Verification items for the finished model (mm, model axes). A direction names the side the tool comes from. Round coordinates to 2 decimals unless told otherwise and drop trailing zeros. Loops run counter-clockwise (first coordinate to the right, second up) from the corner with the lowest first, then second, coordinate; pieces in that order, holes last. Notation, with made-up numbers: M 38.25,36 L 57.25,36 A30 cw 57.25,67 Z; hole C 50,57 d5. An arc over 180 degrees is marked long. Answer as CSV lines item,"result".
Autodesk Inventor part; units mm, degrees
ref_plane "YZ Plane" through (0, 0, 0) normal (1, 0, 0) x (0, 1, 0)
ref_plane "XZ Plane" through (0, 0, 0) normal (0, 1, 0) x (-1, 0, 0)
ref_plane "XY Plane" through (0, 0, 0) normal (0, 0, 1) x (1, 0, 0)
sketch "Sketch1" plane through (0, 0, 0) normal (0, 0, 1) x (1, 0, 0)
  line L0 (0, 0) -> (180, 0)
  line L1 (180, 0) -> (180, -10)
  line L2 (180, -10) -> (0, -10)
  line L3 (0, -10) -> (0, 0)
  line L4 (5.5, 0) -> (24.5, 0)
  line L5 (24.5, 0) -> (24.5, 4.5)
  line L6 (24.5, 4.5) -> (5.5, 4.5)
  line L7 (5.5, 4.5) -> (5.5, 0)
  line L8 (54.5, 4.5) -> (35.5, 4.5)
  line L9 (54.5, 0) -> (54.5, 4.5)
  line L10 (35.5, 4.5) -> (35.5, 0)
  line L11 (84.5, 4.5) -> (65.5, 4.5)
  line L12 (84.5, 0) -> (84.5, 4.5)
  line L13 (65.5, 4.5) -> (65.5, 0)
  line L14 (114.5, 4.5) -> (95.5, 4.5)
  line L15 (114.5, 0) -> (114.5, 4.5)
  line L16 (95.5, 4.5) -> (95.5, 0)
  line L17 (144.5, 4.5) -> (125.5, 4.5)
  line L18 (144.5, 0) -> (144.5, 4.5)
  line L19 (125.5, 4.5) -> (125.5, 0)
  line L20 (174.5, 4.5) -> (155.5, 4.5)
  line L21 (174.5, 0) -> (174.5, 4.5)
  line L22 (155.5, 4.5) -> (155.5, 0)
  dimension "d0" = 180
  dimension "d1" = 10
  dimension "d2" = 19
  dimension "d3" = 4.5
  dimension "d4" = 5.5
  dimension "d7" = 30
extrude "Extrusion1" add sketch "Sketch1" along normal blind 3
properties part number "tray_side_support"
1) Draft check along X on faces 4 (the flat face through (174.5, 2, 1)), 5 (the flat face through (5.5, 2, 1)), 6 (the flat face through (120, 0, 1)). Enter one of: +X half, -X half, draft (parallel to the pull), parting line (faces both ways), or undercut.
Here are the results:
face 4,"+X half"
face 5,"-X half"
face 6,"undercut"
2) Section check C-C (x = 121.5). Record the cut outline in (y, z).
Here are the results:
outline,"M -10,0 L 0,0 L 0,3 L -10,3 Z"
3) Section check A-A (y = 2.5). Record the cut outline in (x, z), plus the area to 3 significant figures.
Here are the results:
outline,"M 5.5,0 L 24.5,0 L 24.5,3 L 5.5,3 Z; M 35.5,0 L 54.5,0 L 54.5,3 L 35.5,3 Z; M 65.5,0 L 84.5,0 L 84.5,3 L 65.5,3 Z; M 95.5,0 L 114.5,0 L 114.5,3 L 95.5,3 Z; M 125.5,0 L 144.5,0 L 144.5,3 L 125.5,3 Z; M 155.5,0 L 174.5,0 L 174.5,3 L 155.5,3 Z"
area,"342 mm^2"
4) Set-up check for faces 1 (the flat face through (45, 4.5, 1)), 2 (the flat face through (177, 0, 1)), 3 (the flat face through (114.5, 2, 1)): record each of +Z, -Z, +X, -X, +Y, -Y from which the full face is reachable in a straight line by a thin tool's end or side.
Here are the results:
face 1,"+Z, -Z, +X, -X, +Y"
face 2,"+Z, -Z, +X, +Y"
face 3,"+Z, -Z, +Y"
5) Go/stop test with flat-tipped pins: pin 1 (0.9 mm diameter, centred on x = 147.5, z = 1.5, fed in from +Y); pin 2 (5 mm diameter, centred on x = 148, y = 3, fed in from +Z); pin 3 (1.5 mm diameter, centred on y = 2.5, z = 1.5, fed in from -X); pin 4 (1.5 mm diameter, centred on y = 2.5, z = 2, fed in from +X). Record where each tip stops, or that it passes through.
Here are the results:
pin 1,"stops at y = 0"
pin 2,"passes through"
pin 3,"stops at x = 5.5"
pin 4,"stops at x = 174.5"
6) Section check B-B (z = 1). Record the cut outline in (x, y).
Here are the results:
outline,"M 0,-10 L 180,-10 L 180,0 L 174.5,0 L 174.5,4.5 L 155.5,4.5 L 155.5,0 L 144.5,0 L 144.5,4.5 L 125.5,4.5 L 125.5,0 L 114.5,0 L 114.5,4.5 L 95.5,4.5 L 95.5,0 L 84.5,0 L 84.5,4.5 L 65.5,4.5 L 65.5,0 L 54.5,0 L 54.5,4.5 L 35.5,4.5 L 35.5,0 L 24.5,0 L 24.5,4.5 L 5.5,4.5 L 5.5,0 L 0,0 Z"
7) Material ranges on probe 1 along X at (y, z) = (3, 2); probe 2 along Y at (x, z) = (124, 1.6), recorded low to high.
Here are the results:
probe 1,"x = 5.5 to 24.5, 35.5 to 54.5, 65.5 to 84.5, 95.5 to 114.5, 125.5 to 144.5, 155.5 to 174.5"
probe 2,"y = -10 to 0"
